Read the model definition and answer for the solid it produces. Units are mm, in the model's axes. Give positions to 0.01 mm unless a question says otherwise; leave off trailing zeros. Loops run counter-clockwise (first coordinate to the right, second up) from the corner with the lowest first, then second, coordinate; pieces in that order, holes last.
(1) Find section B-B, the plane z = 0.5. State how many separate pieces and enclosed holes the cut face has, then the cut area to 3 significant figures.
(2) Find section C-C, the plane x = -39. Write down the section's boundary in (y, z), then the cut area to 4 significant figures.
(3) Each of these flat-tipped pins is pushed along its axis until it touches: P1, Ø0.8, axis at y = 3, z = 0.5, coming from the +X side; P2, Ø0.8, axis at x = -33, z = 1, coming from the -Y side. Where does it stop, or does it pass through?
(4) Straight lines are drawn through the part: probe 1 along Y at (x, z) = (24.5, 0.85); probe 2 along Y at (x, z) = (11.5, 0.75); probe 3 along Y at (x, z) = (-24.5, 0.45). For each, find the intervals that lie inside material, in ascending order.
(5) Find section D-D, the plane y = 21.5. Write down the section's boundary in (x, z), then the cut area to 3 significant figures.
(6) Find section A-A, the plane x = 24.5. Write down the section's boundary in (y, z).
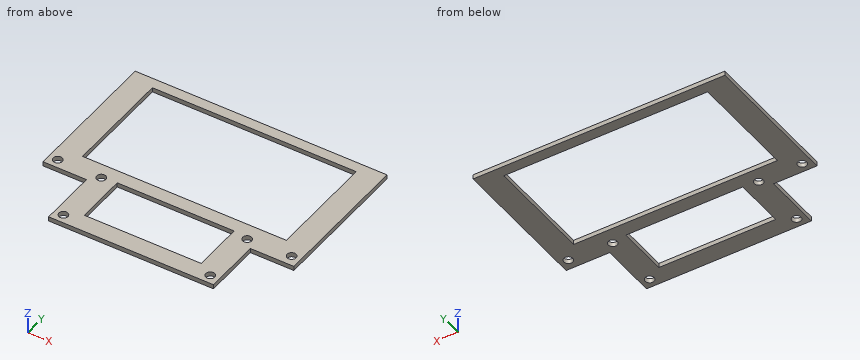
Solid Edge part; units mm, degrees
sketch "Sketch1" plane through (0, 0, 0) normal (0, 0, 1) x (1, 0, 0)
  line L0 (-34, 13.069) -> (34, 13.069)
  line L1 (34, 13.069) -> (34, 49.069)
  line L2 (34, 49.069) -> (-34, 49.069)
  line L3 (-34, 49.069) -> (-34, 13.069)
  line L4 (-19.5, -8.431) -> (19.5, -8.431)
  line L5 (19.5, -8.431) -> (19.5, 8.569)
  line L6 (19.5, 8.569) -> (-19.5, 8.569)
  line L7 (-19.5, 8.569) -> (-19.5, -8.431)
  line L8 (-42, 57.069) -> (-42, 5.069)
  line L9 (-27.5, 5.069) -> (-42, 5.069)
  line L10 (-27.5, -14.431) -> (-27.5, 5.069)
  line L11 (27.5, -14.431) -> (-27.5, -14.431)
  line L12 (27.5, 4.569) -> (27.5, -14.431)
  line L13 (42, 4.569) -> (27.5, 4.569)
  line L14 (42, 57.069) -> (42, 4.569)
  line L15 (-42, 57.069) -> (42, 57.069)
  dimension "D1" = 34
extrude "Protrusion1" add sketch "Sketch1" along normal blind 1.5
sketch "Sketch2" plane through (0, 21.319, 1.5) normal (0, 0, 1) x (0, 1, 0)
  circle A0 centre (-32.75, 24.5) radius 1.5
  circle A1 centre (-32.75, -24.5) radius 1.5
  circle A2 centre (-13.75, -24.5) radius 1.5
  circle A3 centre (-13.25, 24.5) radius 1.5
  circle A4 centre (-13.25, 39) radius 1.5
  circle A5 centre (32.75, 39) radius 1.5
  circle A6 centre (32.75, -39) radius 1.5
  circle A7 centre (-13.25, -39) radius 1.5
  dimension "D1" = 32.75
  dimension "D2" = 32.75
extrude "VaciadoExtruido_29" cut sketch "Sketch2" along normal mid plane 284.5521
sketch "Sketch3" plane through (0, 21.319, 1.5) normal (0, 0, 1) x (0, 1, 0)
  line L0 (31.25, 54.1332) -> (31.25, -56.2447)
  spline S0 degree 3 poles (31.25, 54.1332) (126.4959, 79.9552) (115.951, -69.9426) (31.25, -56.2447) knots 0 0 0 0 1 1 1 1
extrude "VaciadoExtruido_30" cut sketch "Sketch3" along normal mid plane 225.2682
Entries:
1. separate pieces: 1
1. enclosed holes: 8
1. area: 1,920 mm2
2. outline: (5.07, 0) - (6.57, 0) - (6.57, 1.5) - (5.07, 1.5) - close; (9.57, 0) - (52.57, 0) - (52.57, 1.5) - (9.57, 1.5) - close
2. area: 66.75 mm2
3. P1: stops at x = 27.5
3. P2: stops at y = 5.07
4. probe 1: y = -14.43 to -12.93, -9.93 to 6.07, 9.07 to 13.07, 49.07 to 52.57
4. probe 2: y = -14.43 to -8.43, 8.57 to 13.07, 49.07 to 52.57
4. probe 3: y = -14.43 to -12.93, -9.93 to 6.57, 9.57 to 13.07, 49.07 to 52.57
5. outline: (-42, 0) - (-34, 0) - (-34, 1.5) - (-42, 1.5) - close; (34, 0) - (42, 0) - (42, 1.5) - (34, 1.5) - close
5. area: 24.0 mm2
6. outline: (-14.43, 0) - (-12.93, 0) - (-12.93, 1.5) - (-14.43, 1.5) - close; (-9.93, 0) - (6.07, 0) - (6.07, 1.5) - (-9.93, 1.5) - close; (9.07, 0) - (13.07, 0) - (13.07, 1.5) - (9.07, 1.5) - close; (49.07, 0) - (52.57, 0) - (52.57, 1.5) - (49.07, 1.5) - close
